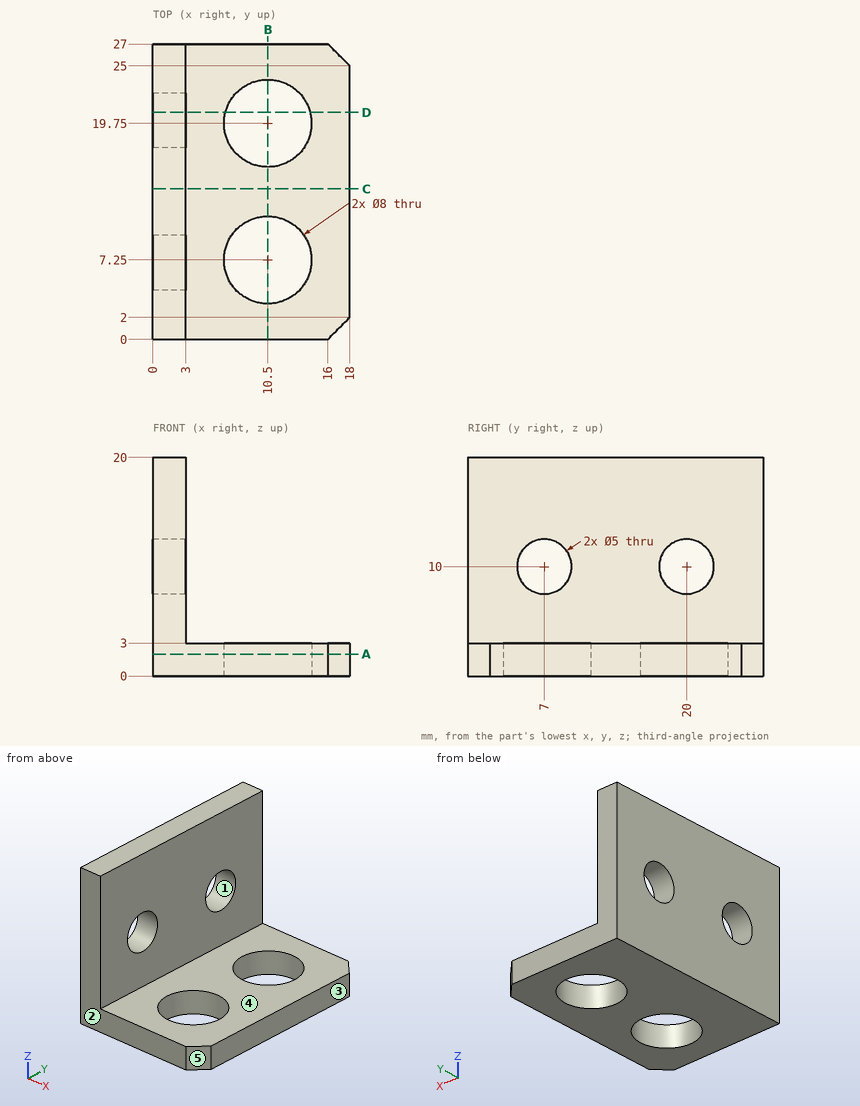
Print and shaded views of the part. All mm, measured from the part's lowest x, y and z. A direction names the side the tool comes from. Coordinates: 2 decimals unless noted, no trailing zeros. Order: outer loops, then holes, each group sorted by start corner. A loop starts at its lowest first (then second) coordinate and runs counter-clockwise, first axis right, second up. Notation, with made-up numbers: (23.5, 18.25) - (28.5, 18.25) arc R26 ccw to (28.5, 55.25) - close; hole circle Ø4 at (48.5, 9). An arc over 180 degrees is marked (long way). Return JSON: item names as keys, results as strings. Group by question number.
Item 1: Pull direction Y, two halves, no side cores. Call the marked faces 1, 2 and 3: pulls with the +Y half, pulls with the -Y half, needs draft (parallel to the pull), parting line crosses it, or undercut.
Item 2: Pin check, flat tips, straight feed: pin 1 (1.5 mm diameter, centred on x = 14, y = 10, fed in from +Z); pin 2 (8.5 mm diameter, centred on y = 18.5, z = 10, fed in from +X). Stop position of each tip, or through.
Item 3: Drill centre lines: probe 1 along Y at (x, z) = (1.8, 10); probe 2 along X at (y, z) = (18.25, 13.5); probe 3 along Y at (x, z) = (1, 8.25). Where is each one in solid material? Low to high. Write a range as from..to.
Item 4: Cut at C-C (y = 13.75). List the corners of the cut face in (x, z).
Item 5: Which spindle directions (+Z, -Z, +X, -X, +Y, -Y) get a long thin tool onto all of the face, cutting with end or side? Do the marked faces 4 and 5. Say none if no direction does.
Item 6: Cut at B-B (x = 10.5). List the corners of the cut face in (y, z).
Item 7: Cut at A-A (z = 2). List the corners of the cut face in (x, y).
Item 8: Cut at D-D (y = 20.75). List the corners of the cut face in (x, z), plus the area to 3 significant figures.
Check values:
{
 "1": {"face 1": "undercut", "face 2": "pulls with the -Y half", "face 3": "needs draft"},
 "2": {"pin 1": "stops at z = 3", "pin 2": "stops at x = 3"},
 "3": {"probe 1": "y = 0..4.5, 9.5..17.5, 22.5..27", "probe 2": "x = 0..3", "probe 3": "y = 0..5.21, 8.79..18.21, 21.79..27"},
 "4": {"outline": "(0, 0) - (18, 0) - (18, 3) - (3, 3) - (3, 20) - (0, 20) - close"},
 "5": {"face 4": "+Z, +X, +Y, -Y", "face 5": "+Z, -Z, +X, -Y"},
 "6": {"outline": "(0, 0) - (3.25, 0) - (3.25, 3) - (0, 3) - close; (11.25, 0) - (15.75, 0) - (15.75, 3) - (11.25, 3) - close; (23.75, 0) - (27, 0) - (27, 3) - (23.75, 3) - close"},
 "7": {"outline": "(0, 0) - (16, 0) - (18, 2) - (18, 25) - (16, 27) - (0, 27) - close; hole circle Ø8 at (10.5, 7.25); hole circle Ø8 at (10.5, 19.75)"},
 "8": {"outline": "(0, 0) - (6.63, 0) - (6.63, 3) - (3, 3) - (3, 7.62) - (0, 7.62) - close; (0, 12.38) - (3, 12.38) - (3, 20) - (0, 20) - close; (14.37, 0) - (18, 0) - (18, 3) - (14.37, 3) - close", "area": "67.5 mm2"}
}
